Source: three-view drawing plus pictorial views. Frame: mm from the lowest corner of the part. Give positions to 0.01 mm unless a question says otherwise; leave off trailing zeros. Order: outer loops, then holes, each group sorted by start corner. A loop starts at its lowest first (then second) coordinate and runs counter-clockwise, first axis right, second up. Notation, with made-up numbers: M -6.75,-9.75 L 51.25,-9.75 A18 ccw 51.25,16.25 Z; hole C 51.25,58.25 d5. An arc over 180 degrees is marked long. Use CSV: the item, a comma, the result in double quotes. Start each with the question number.
1. Pin query (flat end, axial travel): P1, Ø1.5, axis at x = 17, y = 14, coming from the -Z side; P2, Ø5.5, axis at x = 9, y = 12.5, coming from the +Z side; P3, Ø2.5, axis at y = 18, z = 5.5, coming from the -X side; P4, Ø1.5, axis at x = 97.5, z = 41.5, coming from the -Y side. Return the tip coordinate at first contact, or that it passes through.
2. Section query D-D, the plane y = 2.25. Return the cut outline in (x, z).
3. Mould query, pull axis Z, two halves, no side actions, for the marked faces 1, 2, 3 and 4. Classes: released by +Z, released by -Z, zero draft, split by the parting line, or undercut.
4. Section query B-B, the plane x = 9. Return the cut outline in (y, z), plus the area to 4 significant figures.
5. Section query C-C, the plane z = 32.5. Return the cut outline in (x, y), plus the area to 3 significant figures.
6. Section query A-A, the plane y = 12.5. Return the cut outline in (x, z).
7. Line query: line 1 along Y through (x, z) = (9, 50.2); line 2 along Y through (x, z) = (9, 46); line 3 along X through (y, z) = (12.5, 44.65). Output: solid intervals per line, ascending. Write a range as [from, to].
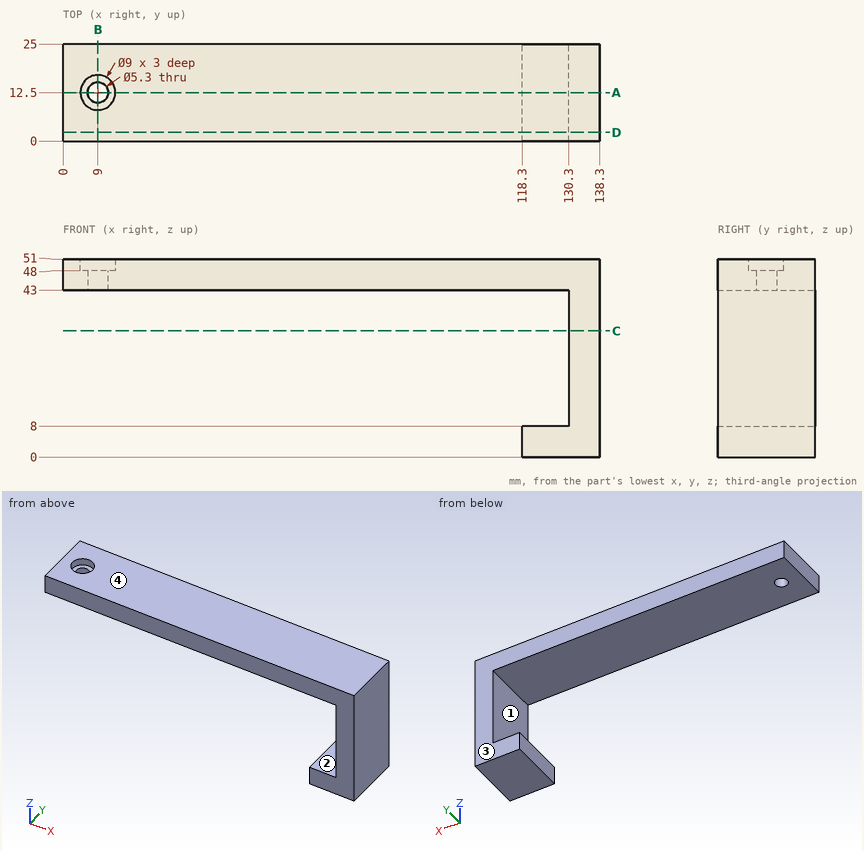
Result set:
1,P1,"z = 43"
1,P2,"z = 48"
1,P3,"x = 118.3"
1,P4,"through"
2,outline,"M 0,43 L 130.3,43 L 130.3,8 L 118.3,8 L 118.3,0 L 138.3,0 L 138.3,51 L 0,51 Z"
3,face 1,"undercut"
3,face 2,"undercut"
3,face 3,"zero draft"
3,face 4,"released by +Z"
4,outline,"M 0,43 L 9.85,43 L 9.85,48 L 8,48 L 8,51 L 0,51 Z; M 15.15,43 L 25,43 L 25,51 L 17,51 L 17,48 L 15.15,48 Z"
4,area,"146.5 mm2"
5,outline,"M 130.3,0 L 138.3,0 L 138.3,25 L 130.3,25 Z"
5,area,"200 mm2"
6,outline,"M 0,43 L 6.35,43 L 6.35,48 L 4.5,48 L 4.5,51 L 0,51 Z; M 11.65,43 L 130.3,43 L 130.3,8 L 118.3,8 L 118.3,0 L 138.3,0 L 138.3,51 L 13.5,51 L 13.5,48 L 11.65,48 Z"
7,line 1,"[0, 8], [17, 25]"
7,line 2,"[0, 9.85], [15.15, 25]"
7,line 3,"[0, 6.35], [11.65, 138.3]"
